from build123d import *

# Parameters (mm, degrees)
BOX003_W     = 136
BOX003_H     = 40
BOX003_DEPTH = 85
BOX002_W     = 20
BOX002_H     = 26.4
BOX002_DEPTH = 100
BOX001_W     = 20
BOX001_H     = 26.4
BOX001_DEPTH = 92
BOX_W        = 170
BOX_H        = 26.4
BOX_DEPTH    = 20
PAD_DEPTH    = 32.4
FILLET_R     = 2
FILLET001_R  = 2
FILLET002_R  = 2
FILLET003_R  = 2
FILLET004_R  = 2


with BuildPart() as cubedessous:
    # Box003 → Box003 (new body)
    with BuildSketch(Plane(origin=(13, -36, -13), x_dir=(1, 0, 0), z_dir=(0, 0, 1))):
        with Locations((68, 20)):
            Rectangle(BOX003_W, BOX003_H)
    extrude(amount=BOX003_DEPTH)


with BuildPart() as cubedroite:
    # Box002 → Box002 (new body)
    with BuildSketch(Plane(origin=(152, -29.4, -11), x_dir=(1, 0, 0), z_dir=(0, 0, 1))):
        with Locations((10, 13.2)):
            Rectangle(BOX002_W, BOX002_H)
    extrude(amount=BOX002_DEPTH)


with BuildPart() as cubegauche:
    # Box001 → Box001 (new body)
    with BuildSketch(Plane(origin=(-10, -29.4, -4), x_dir=(1, 0, 0), z_dir=(0, 0, 1))):
        with Locations((10, 13.2)):
            Rectangle(BOX001_W, BOX001_H)
    extrude(amount=BOX001_DEPTH)


with BuildPart() as cubedessus:
    # Box → Box (new body)
    with BuildSketch(Plane(origin=(-4, -29.4, 75), x_dir=(1, 0, 0), z_dir=(0, 0, 1))):
        with Locations((85, 13.2)):
            Rectangle(BOX_W, BOX_H)
    extrude(amount=BOX_DEPTH)


with BuildPart() as fillet004:
    # Sketch → Pad (new body)
    with BuildSketch(Plane.XZ):
        with BuildLine():
            ThreePointArc((5, 85), (1.464466, 83.535534), (0, 80))
            Line((0, 0), (0, 80))
            Line((0, 0), (162, 0))
            Line((162, 80), (162, 0))
            ThreePointArc((162, 80), (160.535534, 83.535534), (157, 85))
            Line((5, 85), (157, 85))
        make_face()
    extrude(amount=PAD_DEPTH)

    # Cut: cut CubeDessus
    add(cubedessus.part, mode=Mode.SUBTRACT)

    # Cut001: cut CubeGauche
    add(cubegauche.part, mode=Mode.SUBTRACT)

    # Cut002: cut CubeDroite
    add(cubedroite.part, mode=Mode.SUBTRACT)

    # Cut003: cut CubeDessous
    add(cubedessous.part, mode=Mode.SUBTRACT)

    # Fillet
    fillet_edges = [fillet004.edges().sort_by_distance(p)[0] for p in [
        (152, -16.2, 75),
    ]]
    fillet(fillet_edges, radius=FILLET_R)

    # Fillet001
    fillet001_edges = [fillet004.edges().sort_by_distance(p)[0] for p in [
        (10, -16.2, 75),
    ]]
    fillet(fillet001_edges, radius=FILLET001_R)

    # Fillet002
    fillet002_edges = [fillet004.edges().sort_by_distance(p)[0] for p in [
        (81, -32.4, 85),
        (1.464466, -32.4, 83.535534),
        (0, -32.4, 40),
        (162, -32.4, 40),
        (160.535534, -32.4, 83.535534),
    ]]
    fillet(fillet002_edges, radius=FILLET002_R)

    # Fillet003
    fillet003_edges = [fillet004.edges().sort_by_distance(p)[0] for p in [
        (1.464466, 0, 83.535534),
        (0, 0, 40),
        (162, 0, 40),
        (160.535534, 0, 83.535534),
        (81, 0, 85),
    ]]
    fillet(fillet003_edges, radius=FILLET003_R)

    # Fillet004
    fillet004_edges = [fillet004.edges().sort_by_distance(p)[0] for p in [
        (13, -16.2, 72),
        (149, -16.2, 72),
    ]]
    fillet(fillet004_edges, radius=FILLET004_R)


solid = fillet004.part
Verification items for the finished model (mm, model axes). A direction names the side the tool comes from. Coordinates: 2 decimals unless noted, no trailing zeros. Write each loop counter-clockwise with the first axis right and the second up, starting at its lowest first coordinate (ties: lowest second). Pieces come first, ordered by that corner, then holes. Notation, with made-up numbers: (67.25, 32) -> (121.25, 32) arc R16 ccw to (121.25, 41) -> close; hole circle Ø2 at (-20, 32). An arc over 180 degrees is marked (long way). One line per item, written item: value. Start each with the question number.
Q1. Go/stop test with flat-tipped pins: P1, Ø13, axis at y = -21.5, z = 27, coming from the +X side; P2, Ø13, axis at y = -10, z = 26.5, coming from the -X side; P3, Ø3, axis at x = 45, y = -6.5, coming from the +Z side. Record where each tip stops, or that it passes through.
Q2. Access from +Z, -Z, +X, -X, +Y, -Y to the whole of each face (thin tool, end or side, straight path). Record for faces 1 (the flat face through (80, -16, 72)), 2 (the flat face through (152, -16, 36)), 3 (the flat face through (80, -16, 75)), 4 (the flat face through (87, -3, 77)), 5 (the flat face through (10, -16, 36)).
Q3. Cross-section at A-A on z = 7. Enter the section's corners in (x, y).
Q4. Thickness scan on L1, parallel to X at y = -27, z = 5.5; L2, parallel to Y at x = 28.5, z = 77.5; L3, parallel to X at y = -2.5, z = 30.5. Record the ranges inside material, lowest first. Write a range as from..to.
Q5. Cross-section at B-B on y = -9.5. Enter the section's corners in (x, z).
Q6. Cross-section at C-C on x = 63. Enter the section's corners in (y, z).
Q7. Mould release check, pull along Y, two halves, no side actions. Record for faces 6 (the flat face through (80.6, -32.4, 72.4)), 7 (the flat face through (11, -16, 0)), 8 (the flat face through (87, -29.4, 77)): pulls with the +Y half, pulls with the -Y half, needs draft (parallel to the pull), parting line crosses it, or undercut.
Checked values:
1. P1: stops at x = 152
1. P2: stops at x = 10
1. P3: stops at z = 75
2. face 1: -Z, +Y, -Y
2. face 2: +Z, -Z, +X
2. face 3: +Z, +X, -X
2. face 4: +Z
2. face 5: +Z, -Z, -X
3. outline: (0, -30.4) arc R2 ccw to (2, -32.4) -> (13, -32.4) -> (13, 0) -> (2, 0) arc R2 ccw to (0, -2) -> (0, -3) -> (10, -3) -> (10, -29.4) -> (0, -29.4) -> close; (149, -32.4) -> (160, -32.4) arc R2 ccw to (162, -30.4) -> (162, -29.4) -> (152, -29.4) -> (152, -3) -> (162, -3) -> (162, -2) arc R2 ccw to (160, 0) -> (149, 0) -> close
4. L1: x = 10..13, 149..152
4. L2: y = -32.4..-29.4, -3..0
4. L3: x = 0..13, 149..162
5. outline: (10, 0) -> (13, 0) -> (13, 70) arc R2 cw to (15, 72) -> (147, 72) arc R2 cw to (149, 70) -> (149, 0) -> (152, 0) -> (152, 73) arc R2 ccw to (150, 75) -> (12, 75) arc R2 ccw to (10, 73) -> close
6. outline: (-32.4, 72) -> (0, 72) -> (0, 83) arc R2 ccw to (-2, 85) -> (-3, 85) -> (-3, 75) -> (-29.4, 75) -> (-29.4, 85) -> (-30.4, 85) arc R2 ccw to (-32.4, 83) -> close
7. face 6: pulls with the -Y half
7. face 7: needs draft
7. face 8: undercut
